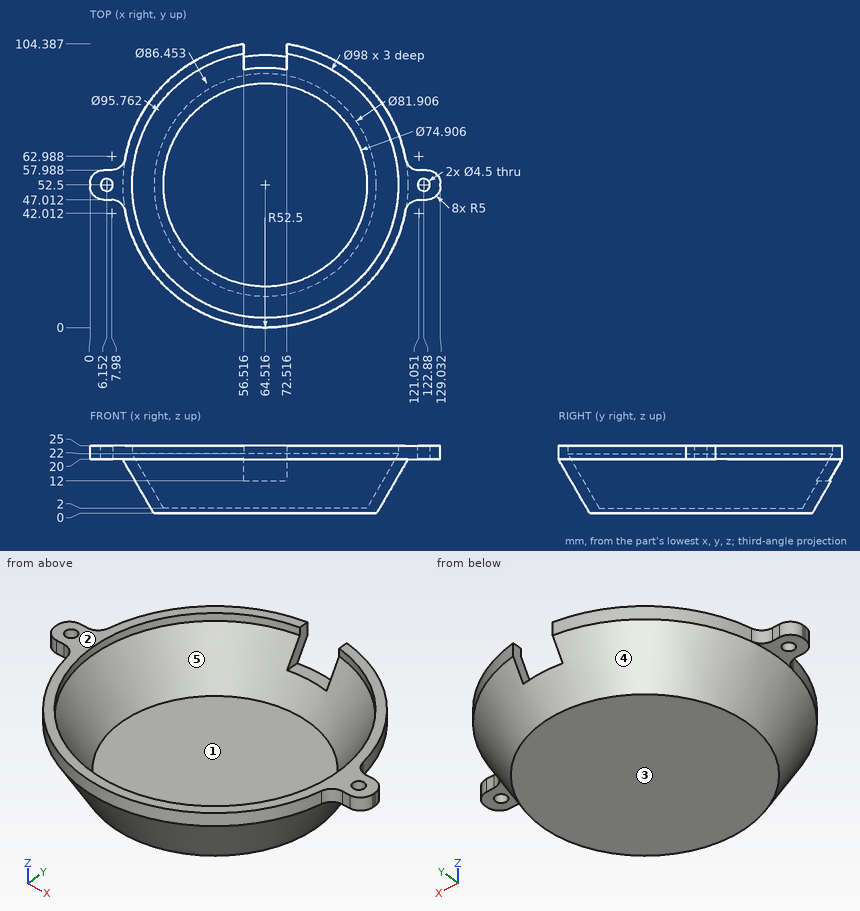
Job drawing, mm, ordinate dimensions from the low corner. One solid piece. A direction names the side the tool comes from. Coordinates: 2 decimals unless noted, no trailing zeros. Answer as a JSON object with one key per item and string values. Group by question number.
(1) Flat gauge pins, fed straight in: pin 1 (2.5 mm diameter, centred on x = 122, z = 23, fed in from +Y); pin 2 (6 mm diameter, centred on x = 93.5, y = 54, fed in from +Z); pin 3 (4.5 mm diameter, centred on x = 65, y = 97.5, fed in from +Z); pin 4 (3.5 mm diameter, centred on x = 6.15, y = 52.5, fed in from -Z). Where does each tip first touch, or does it go through?
(2) Tool access for the marked faces 1 and 2: list every direction of +Z, -Z, +X, -X, +Y, -Y with a clear straight run to the whole face (end or side of a thin tool).
(3) Probe line 1 along Z through (x, y) = (85.5, 25.5); line 2 along Y through (x, z) = (83.5, 13) (1 decimal); line 3 along Y through (x, z) = (80, 3.25) (1 decimal). List the from-to ranges inside material, lowest first.
(4) Two-plate mould, pull along X, no slides. Class the marked faces 3, 4 and 5: released by +X, released by -X, zero draft, split by the parting line, or undercut.
Geometry says:
{
 "1": {"pin 1": "stops at y = 58", "pin 2": "stops at z = 2", "pin 3": "stops at z = 12", "pin 4": "passes through"},
 "2": {"face 1": "+Z", "face 2": "+Z, +X, -X, +Y, -Y"},
 "3": {"line 1": "z = 0 to 2", "line 2": "y = 7.9 to 13, 92 to 97.1", "line 3": "y = 12.6 to 17.6, 87.4 to 92.4"},
 "4": {"face 3": "zero draft", "face 4": "split by the parting line", "face 5": "undercut"}
}
